For this review, take the finished solid that the model builds, in its own axes (mm). Give positions to 0.01 mm unless a question says otherwise; leave off trailing zeros. Order: outer loops, then holes, each group sorted by start corner. A loop starts at its lowest first (then second) coordinate and runs counter-clockwise, first axis right, second up. Notation, with made-up numbers: (20, 77.5) -> (27, 77.5) arc R30 cw to (27, 100.5) -> close; hole circle Ø2 at (-31.5, 15.25). An arc over 180 degrees is marked (long way). One line per item, written item: value. Start each with the question number.
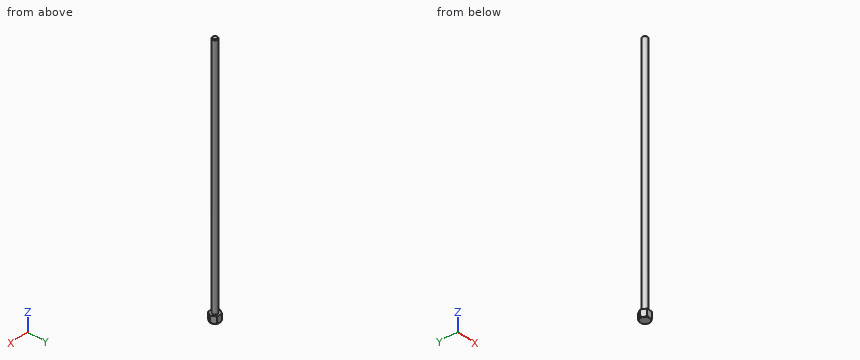
from build123d import *

# Parameters (mm, degrees)
F0_R     = 2.5
F0_R_2   = 1.9
F1_DEPTH = 5
F2_DEPTH = 179
F7_SIZE  = 0.5


with BuildPart() as f1:
    # F0 (on Top) → F1 (new body)
    with BuildSketch(Plane.XY):
        Polygon((3.75, 0), (1.875, 3.247595), (-1.875, 3.247595), (-3.75, 0), (-1.875, -3.247595), (1.875, -3.247595), align=None)
        Circle(F0_R, mode=Mode.SUBTRACT)
        Circle(F0_R)
        Circle(F0_R_2, mode=Mode.SUBTRACT)
    extrude(amount=F1_DEPTH)

    # F0 (on Top) → F2 (join)
    with BuildSketch(Plane.XY):
        Circle(F0_R_2)
    extrude(amount=F2_DEPTH)

    # F5 (on Front) → F6 (revolve, cut)
    with BuildSketch(Plane.XZ):
        Polygon((3.75, 1), (3.247595, 0), (3.75, 0), align=None)
    revolve(axis=Axis((0, 0, 1.934983), (0, 0, 1)), mode=Mode.SUBTRACT)

    # F7
    f7_edges = [f1.edges().sort_by_distance(p)[0] for p in [
        (-1.9, 0, 179),
    ]]
    chamfer(f7_edges, length=F7_SIZE)


solid = f1.part
Q1. For line 1 along Z through (x, y) = (-1.75, -1.25); line 2 along Y through (x, z) = (0, 169); line 3 along X through (y, z) = (0.25, 74), list the stretches that pass through material, from the lowest coordinate up.
Q2. Take a section at A-A (z = 56.5). State the section outline as (x, y) points.
Q3. For pin 1 Ø1 at (y, z) = (-1.5, 26) entering from +X; pin 2 Ø1 at (x, z) = (1, 130) entering from -Y; pin 3 Ø1 at (x, z) = (-1.5, 79) entering from +Y, all flat-tipped, find the tip position at first contact; note any pin that passes through.
Answers below:
1. line 1: z = 0 to 5
1. line 2: y = -1.9 to 1.9
1. line 3: x = -1.88 to 1.88
2. outline: circle Ø3.8 at (0, 0)
3. pin 1: stops at x = 1.62
3. pin 2: stops at y = -1.83
3. pin 3: stops at y = 1.62
